from build123d import *

# Parameters (mm, degrees)
SKETCH1_W            = 24
SKETCH1_H            = 15
BOSS_EXTRUDE1_DEPTH  = 0.75
BOSS_EXTRUDE2_START  = -1.5
BOSS_EXTRUDE2_DEPTH  = 4
MIRROR2_START        = -1.5
MIRROR2_COPY_1_DEPTH = 4
FILLET1_R            = 1


with BuildPart() as part:
    # Sketch1 → Boss-Extrude1 (new, symmetric)
    with BuildSketch(Plane(origin=(0, 0, 0), x_dir=(1, 0, 0), z_dir=(0, 1, 0))):
        Rectangle(SKETCH1_W, SKETCH1_H)
    extrude(amount=BOSS_EXTRUDE1_DEPTH, both=True)

    # Sketch2 → Boss-Extrude2 (add)
    with BuildSketch(Plane(origin=(0, 0.75, 0), x_dir=(1, 0, 0), z_dir=(0, 1, 0)).offset(BOSS_EXTRUDE2_START)):
        Polygon((-12, 4.5), (-14, 4.5), (-14, 9.5), (-9, 9.5), (-9, 7.5), (-12, 7.5), align=None)
    boss_extrude2 = extrude(amount=BOSS_EXTRUDE2_DEPTH)

    # Mirror1: Boss-Extrude2 across plane
    add(boss_extrude2.mirror(Plane(origin=(0, 0, 0), x_dir=(0, 0, 1), z_dir=(1, 0, 0))))

    # Mirror2: Boss-Extrude2 across plane
    add(boss_extrude2.mirror(Plane.XY))

    # Mirror2 copy 1 sketch → Mirror2 copy 1 (add)
    with BuildSketch(Plane(origin=(0, 0.75, 0), x_dir=(-1, 0, 0), z_dir=(0, 1, 0)).offset(MIRROR2_START)):
        Polygon((-12, 4.5), (-14, 4.5), (-14, 9.5), (-9, 9.5), (-9, 7.5), (-12, 7.5), align=None)
    extrude(amount=MIRROR2_COPY_1_DEPTH)

    # Fillet1
    fillet1_edges = [part.edges().sort_by_distance(p)[0] for p in [
        (12, 0.75, 6),
        (-10.5, 0.75, -7.5),
        (10.5, 0.75, -7.5),
        (-14, 1.25, -9.5),
        (-11.5, 3.25, -9.5),
        (-14, 3.25, -7),
        (12, 0.75, -6),
        (11.5, 3.25, -9.5),
        (14, 1.25, -9.5),
        (14, 3.25, -7),
        (-12, 0.75, -6),
        (-12, 0.75, 6),
        (-11.5, 3.25, 9.5),
        (-14, 1.25, 9.5),
        (-14, 3.25, 7),
        (10.5, 0.75, 7.5),
        (14, 1.25, 9.5),
        (11.5, 3.25, 9.5),
        (14, 3.25, 7),
        (-10.5, 0.75, 7.5),
    ]]
    fillet(fillet1_edges, radius=FILLET1_R)


solid = part.part
Source: CAD feature listing. Evaluate the final solid. Frame: model axes, mm. A direction names the side the tool comes from. Round coordinates to 2 decimals unless told otherwise and drop trailing zeros. Loops run counter-clockwise (first coordinate to the right, second up) from the corner with the lowest first, then second, coordinate; pieces in that order, holes last.
Q1. Ray query, line 1 (X direction, y = 1.4, z = 8.25); line 2 (Z direction, x = 12.5, y = 0.9); line 3 (X direction, y = 1.9, z = -6.5). Return the intervals inside material, ascending.
Q2. Section D-D, the plane z = 3.25. Return loops of the section in (x, y), plus the area to 3 significant figures.
Q3. Section A-A, the plane y = 1.05. Return loops of the section in (x, z), plus the area to 3 significant figures.
Q4. Access query for faces 4 (the face through (10.521, 1.035, -7.199)), 5 (the face through (13.715, 0.771, -9.199)), 6 (the face through (12, 0, 0)), 7 (the face through (-12, 0, 0)), 8 (the face through (-14, 1, -6)). Directions: +Z, -Z, +X, -X, +Y, -Y. A direction counts if a zero-diameter tool reaches every point of the face in a straight line with its end or side. Return the directions, or none.
Q5. Mould query, pull axis Z, two halves, no side actions, for faces 1 (the face through (-13.699, 0.771, -9.215)), 2 (the face through (-13, 1, -4.5)), 3 (the face through (12, 3.25, -8)). Classes: pulls with the +Z half, pulls with the -Z half, needs draft (parallel to the pull), parting line crosses it, or undercut.
Q6. Section B-B, the plane z = -6. Return loops of the section in (x, y), plus the area to 3 significant figures.
Q7. First-contact query: P1, Ø1.2, axis at x = -3, y = 0, coming from the -Z side; P2, Ø8, axis at x = -5.5, z = 3, coming from the +Y side; P3, Ø1.2, axis at y = 0, z = 0.5, coming from the -X side. Flat tips, straight axial feed; report the tip coordinate or a pass-through.
Q8. Section C-C, the plane x = 0.75. Return loops of the section in (y, z), plus the area to 3 significant figures.
Solutions:
1. line 1: x = -14 to -9, 9 to 14
1. line 2: z = -9.5 to -4.5, 4.5 to 9.5
1. line 3: x = -14 to -12, 12 to 14
2. outline: (-12, -0.75) - (12, -0.75) - (12, 0.75) - (-12, 0.75) - close
2. area: 36.0 mm2
3. outline: (-14, -8.5) arc R1 ccw to (-13, -9.5) - (-9, -9.5) - (-9, -7.21) - (-11.71, -7.21) - (-11.71, -4.5) - (-14, -4.5) - close; (-14, 4.5) - (-11.71, 4.5) - (-11.71, 7.21) - (-9, 7.21) - (-9, 9.5) - (-13, 9.5) arc R1 ccw to (-14, 8.5) - close; (9, -9.5) - (13, -9.5) arc R1 ccw to (14, -8.5) - (14, -4.5) - (11.71, -4.5) - (11.71, -7.21) - (9, -7.21) - close; (9, 7.21) - (11.71, 7.21) - (11.71, 4.5) - (14, 4.5) - (14, 8.5) arc R1 ccw to (13, 9.5) - (9, 9.5) - close
3. area: 69.7 mm2
4. face 4: +Y
4. face 5: -Z, +X, +Y, -Y
4. face 6: +X, +Y, -Y
4. face 7: -X, +Y, -Y
4. face 8: +Z, -Z, -X, +Y, -Y
5. face 1: pulls with the -Z half
5. face 2: undercut
5. face 3: needs draft
6. outline: (-14, -0.75) - (14, -0.75) - (14, 2.25) arc R1 ccw to (13, 3.25) - (12, 3.25) - (12, 1.75) arc R1 cw to (11, 0.75) - (-11, 0.75) arc R1 cw to (-12, 1.75) - (-12, 3.25) - (-13, 3.25) arc R1 ccw to (-14, 2.25) - close
6. area: 52.0 mm2
7. P1: stops at z = -7.5
7. P2: stops at y = 0.75
7. P3: stops at x = -12
8. outline: (-0.75, -7.5) - (0.75, -7.5) - (0.75, 7.5) - (-0.75, 7.5) - close
8. area: 22.5 mm2
